```python
from build123d import *

# Parameters (mm, degrees)
F0_W     = 540
F0_H     = 390
F1_DEPTH = 10
F2_W     = 80
F2_H     = 80
F2_R     = 15
F3_DEPTH = 10
F5_W     = 380
F5_H     = 80
F6_DEPTH = 10
F7_DEPTH = 25
F8_W     = 111.767
F8_H     = 26.2346411405
F9_DEPTH = 25


with BuildPart() as f1:
    # F0 (on Front) → F1 (new body)
    with BuildSketch(Plane.XZ):
        Polygon((-575.5810141563, 243.9473703504), (-465.5810141563, -206.0526296496), (133.660423523, -206.0526296496), (243.660423523, 243.9473703504), (133.660423523, 243.9473703504), (-465.5810141563, 243.9473703504), align=None)
        with Locations((-166.339576477, 18.9473703504)):
            Rectangle(F0_W, F0_H, mode=Mode.SUBTRACT)
        Polygon((-495.5810141563, 43.0153865893), (-537.3643879646, 213.9473703504), (-495.5810141563, 213.9473703504), align=None, mode=Mode.SUBTRACT)
        Polygon((163.660423523, 213.9473703504), (205.4437973313, 213.9473703504), (163.660423523, 43.0153865893), align=None, mode=Mode.SUBTRACT)
    extrude(amount=F1_DEPTH)

    # F2 (on face) → F3 (join)
    with BuildSketch(Plane.XZ.offset(10)):
        with Locations((-396.339576477, 173.9473703504)):
            Rectangle(F2_W, F2_H)
        with Locations((-396.339576477, 173.9473703504)):
            Circle(F2_R, mode=Mode.SUBTRACT)
        with Locations((63.660423523, 173.9473703504)):
            Rectangle(F2_W, F2_H)
        with Locations((63.660423523, 173.9473703504)):
            Circle(F2_R, mode=Mode.SUBTRACT)
        with Locations((63.660423523, -136.0526296496)):
            Rectangle(F2_W, F2_H)
        with Locations((63.660423523, -136.0526296496)):
            Circle(F2_R, mode=Mode.SUBTRACT)
        with Locations((-396.339576477, -136.0526296496)):
            Rectangle(F2_W, F2_H)
        with Locations((-396.339576477, -136.0526296496)):
            Circle(F2_R, mode=Mode.SUBTRACT)
    extrude(amount=-F3_DEPTH)

    # F5 (on face) → F6 (join)
    with BuildSketch(Plane.XZ.offset(10)):
        with Locations((-166.339576477, 173.9473703504)):
            Rectangle(F5_W, F5_H)
    extrude(amount=-F6_DEPTH)

    # F4 (on face) → F7 (cut)
    with BuildSketch(Plane.XZ.offset(10)):
        Polygon((3.5932296524, 243.9473703504), (-339.0040903476, 243.9473703504), (-339.0040903476, 218.5033703504), (-286.9719266891, 218.5033703504), (3.5932296524, 218.5033703504), align=None)
    extrude(amount=-F7_DEPTH, mode=Mode.SUBTRACT)

    # F8 (on face) → F9 (cut)
    with BuildSketch(Plane.XZ.offset(10)):
        with Locations((-193.0365383425, 205.3860497801)):
            Rectangle(F8_W, F8_H)
    extrude(amount=-F9_DEPTH, mode=Mode.SUBTRACT)


solid = f1.part
```
Could you check a few things on this model? Use its own coordinates, in mm. Give positions to 0.01 mm unless a question says otherwise; leave off trailing zeros. Loops run counter-clockwise (first coordinate to the right, second up) from the corner with the lowest first, then second, coordinate; pieces in that order, holes last. Notation, with made-up numbers: (50, -6.75) - (106, -6.75) arc R20 cw to (106, 0.25) - close; hole circle Ø10 at (30, 72.25). An arc over 180 degrees is marked (long way). Use one line per item in the form item = value.
1. I need wall thicknesses on probe 1 along Z at (x, y) = (-72.5, -6); probe 2 along Z at (x, y) = (-367.5, -5.75); probe 3 along X at (y, z) = (-2.25, 220.5). Which ranges of each line are inside material? Lowest first, please.
Response values:
probe_1 = -206.05 to -176.05, 133.95 to 218.5
probe_2 = -206.05 to -96.05, 133.95 to 243.95
probe_3 = -569.85 to -339, 3.59 to 237.93
2. Thinking about a two-plate mould opening in Z: for faces 1 (the face through (-411.325, -5.07, -135.393)), 2 (the face through (-521.35, -4.93, 22.1)), 3 (the face through (-172, 0, 172)), which applies, released by +Z, released by -Z, zero draft, split by the parting line, or undercut?
Response values:
face_1 = undercut
face_2 = released by -Z
face_3 = zero draft
3. I want a section at D-D (z = -73.5). Please give me the cut outline in (x, y), and give its area (3 significant figures).
Response values:
outline = (-497.98, -10) - (-436.34, -10) - (-436.34, 0) - (-497.98, 0) - close; (103.66, -10) - (166.06, -10) - (166.06, 0) - (103.66, 0) - close
area = 1,240 mm²
4. I want a section at A-A (x = -170). Please give me the cut outline in (y, z).
Response values:
outline = (-10, -206.05) - (0, -206.05) - (0, -176.05) - (-10, -176.05) - close; (-10, 133.95) - (0, 133.95) - (0, 192.27) - (-10, 192.27) - close
5. I'm going to push flat-ended pins straight in: pin 1 Ø5 at (x, y) = (-190, -6) entering from +Z; pin 2 Ø3 at (y, z) = (-3, 55) entering from -X; pin 3 Ø24 at (x, z) = (-396.34, 173.95) entering from -Y; pin 4 Ø1.5 at (x, y) = (2, -4) entering from +Z. Where does each tip first touch, or does it pass through?
Response values:
pin_1 = 192.27
pin_2 = -529.76
pin_3 = through
pin_4 = 218.5
6. I want a section at B-B (z = 97). Please give me the cut outline in (x, y), and give its area (3 significant figures).
Response values:
outline = (-539.66, -10) - (-508.78, -10) - (-508.78, 0) - (-539.66, 0) - close; (-495.58, -10) - (-436.34, -10) - (-436.34, 0) - (-495.58, 0) - close; (103.66, -10) - (163.66, -10) - (163.66, 0) - (103.66, 0) - close; (176.86, -10) - (207.74, -10) - (207.74, 0) - (176.86, 0) - close
area = 1,810 mm²
7. I want a section at C-C (y = -1.5). Give the number of separate pieces and of enclosed holes in the cut face, and give its area (3 significant figures).
Response values:
separate_pieces = 1
enclosed_holes = 7
area = 143,000 mm²
